Part model, mm, in its own coordinate system. Face numbers are marked on the shaded views. A direction names the side the tool comes from. Coordinates: 2 decimals unless noted, no trailing zeros. Order: outer loops, then holes, each group sorted by start corner. A loop starts at its lowest first (then second) coordinate and runs counter-clockwise, first axis right, second up.
1) Wall check: L1, parallel to Z at x = -18, y = 19.75; L2, parallel to X at y = 11.25, z = 20; L3, parallel to X at y = 20.1, z = -20. Give the ranges that are in metal, low to high.
2) Cut at C-C (z = 14). List the corners of the cut face in (x, y), and give its area (3 significant figures).
3) Pin check, flat tips, straight feed: pin 1 Ø2 at (y, z) = (18, -5.5) entering from +X; pin 2 Ø3.5 at (x, y) = (-0.5, 16) entering from -Z; pin 3 Ø4.5 at (x, z) = (18, 0.5) entering from +Y. Stop position of each tip, or through.
4) Mould opens along Z. For the marked faces 1, 2 and 3 say: +Z half, -Z half, draft (parallel to the pull), parting line (faces both ways), or undercut.
5) Cut at A-A (z = 1). List the corners of the cut face in (x, y), and give its area (3 significant figures).
6) Cut at D-D (x = 14.5). List the corners of the cut face in (y, z).
7) Cut at B-B (y = 9.25). List the corners of the cut face in (x, z), and give its area (3 significant figures).
8) Tool access for the marked faces 4, 5 and 6: list every direction of +Z, -Z, +X, -X, +Y, -Y with a clear straight run to the whole face (end or side of a thin tool).
```python
from build123d import *

# Parameters (mm, degrees)
ESQUISSE1_R             = 1.5
BOSS_EXTRU_1_DEPTH      = 20
ESQUISSE2_R             = 2.25
ESQUISSE2_R_2           = 1.5
BOSS_EXTRU_2_DEPTH      = 1.5
ESQUISSE6_W             = 7.215685205
ESQUISSE6_H             = 18.365547593
ESQUISSE6_W_2           = 15.795882497
ESQUISSE6_H_2           = 7.128539117
ESQUISSE6_W_3           = 6.98895005
ESQUISSE6_H_3           = 20.179428837
BOSS_EXTRU_3_DEPTH      = 14.8
ENL_V_MAT_EXTRU_1_DEPTH = 20
ENL_V_MAT_EXTRU_1_DRAFT = 10
ENL_V_MAT_EXTRU_2_DEPTH = 20
ENL_V_MAT_EXTRU_2_DRAFT = 7
ESQUISSE5_R             = 2.5
ENL_V_MAT_EXTRU_3_DEPTH = 18
CONG_4_R                = 1
CONG_5_R                = 1
CONG_6_R                = 1
CONG_7_R                = 1


with BuildPart() as part:
    # Esquisse1 → Boss.-Extru.1 (new body)
    with BuildSketch(Plane(origin=(0, 0, 0), x_dir=(1, 0, 0), z_dir=(0, 1, 0))):
        with BuildLine():
            Line((-19, 4.2), (-17.6, 4.2))
            ThreePointArc((-17.6, 4.2), (-15.832233047, 3.467766953), (-15.1, 1.7))
            Line((-15.1, 1.7), (-15.1, -1.7))
            ThreePointArc((-15.1, -1.7), (-15.832233047, -3.467766953), (-17.6, -4.2))
            Line((-17.6, -4.2), (-19, -4.2))
            ThreePointArc((-19, -4.2), (-20.767766953, -4.932233047), (-21.5, -6.7))
            Line((-21.5, -6.7), (-21.5, -20.5))
            Line((-21.5, -20.5), (-21.5, -23))
            Line((-21.5, -23), (-19, -23))
            Line((-19, -23), (-6.7, -23))
            ThreePointArc((-6.7, -23), (-4.932233047, -22.267766953), (-4.2, -20.5))
            Line((-4.2, -20.5), (-4.2, -19.1))
            ThreePointArc((-4.2, -19.1), (-3.467766953, -17.332233047), (-1.7, -16.6))
            Line((-1.7, -16.6), (1.7, -16.6))
            ThreePointArc((1.7, -16.6), (3.467766953, -17.332233047), (4.2, -19.1))
            Line((4.2, -19.1), (4.2, -20.5))
            ThreePointArc((4.2, -20.5), (4.932233047, -22.267766953), (6.7, -23))
            Line((6.7, -23), (19, -23))
            Line((19, -23), (21.5, -23))
            Line((21.5, -23), (21.5, -20.5))
            Line((21.5, -20.5), (21.5, -6.7))
            ThreePointArc((21.5, -6.7), (20.767766953, -4.932233047), (19, -4.2))
            Line((19, -4.2), (17.6, -4.2))
            ThreePointArc((17.6, -4.2), (15.832233047, -3.467766953), (15.1, -1.7))
            Line((15.1, -1.7), (15.1, 1.7))
            ThreePointArc((15.1, 1.7), (15.832233047, 3.467766953), (17.6, 4.2))
            Line((17.6, 4.2), (19, 4.2))
            ThreePointArc((19, 4.2), (20.767766953, 4.932233047), (21.5, 6.7))
            Line((21.5, 6.7), (21.5, 20.5))
            Line((21.5, 20.5), (21.5, 23))
            Line((21.5, 23), (19, 23))
            Line((19, 23), (6.7, 23))
            ThreePointArc((6.7, 23), (4.932233047, 22.267766953), (4.2, 20.5))
            Line((4.2, 20.5), (4.2, 19.1))
            ThreePointArc((4.2, 19.1), (3.467766953, 17.332233047), (1.7, 16.6))
            Line((1.7, 16.6), (-1.7, 16.6))
            ThreePointArc((-1.7, 16.6), (-3.467766953, 17.332233047), (-4.2, 19.1))
            Line((-4.2, 19.1), (-4.2, 20.5))
            ThreePointArc((-4.2, 20.5), (-4.932233047, 22.267766953), (-6.7, 23))
            Line((-6.7, 23), (-19, 23))
            Line((-19, 23), (-21.5, 23))
            Line((-21.5, 23), (-21.5, 20.5))
            Line((-21.5, 20.5), (-21.5, 6.7))
            ThreePointArc((-21.5, 6.7), (-20.767766953, 4.932233047), (-19, 4.2))
        make_face()
        with Locations(Location((-18, 20, 0), (0, 0, 270))):
            Circle(ESQUISSE1_R, mode=Mode.SUBTRACT)
        with Locations(Location((18, 20, 0), (0, 0, 270))):
            Circle(ESQUISSE1_R, mode=Mode.SUBTRACT)
        with Locations(Location((18, -20, 0), (0, 0, 270))):
            Circle(ESQUISSE1_R, mode=Mode.SUBTRACT)
        with Locations(Location((-18, -20, 0), (0, 0, 270))):
            Circle(ESQUISSE1_R, mode=Mode.SUBTRACT)
    extrude(amount=BOSS_EXTRU_1_DEPTH)

    # Esquisse2 → Boss.-Extru.2 (add)
    # profile 1 of 4: a face of its own
    with BuildSketch(Plane(origin=(0, 20, 0), x_dir=(1, 0, 0), z_dir=(0, 1, 0))):
        with Locations(Location((-18, 20, 0), (0, 0, 270))):
            Circle(ESQUISSE2_R)
        with Locations(Location((-18, 20, 0), (0, 0, 270))):
            Circle(ESQUISSE2_R_2, mode=Mode.SUBTRACT)
    # profile 2 of 4: a face of its own
    with BuildSketch(Plane(origin=(0, 20, 0), x_dir=(1, 0, 0), z_dir=(0, 1, 0))):
        with Locations(Location((18, 20, 0), (0, 0, 270))):
            Circle(ESQUISSE2_R)
        with Locations(Location((18, 20, 0), (0, 0, 270))):
            Circle(ESQUISSE2_R_2, mode=Mode.SUBTRACT)
    # profile 3 of 4: a face of its own
    with BuildSketch(Plane(origin=(0, 20, 0), x_dir=(1, 0, 0), z_dir=(0, 1, 0))):
        with Locations(Location((18, -20, 0), (0, 0, 270))):
            Circle(ESQUISSE2_R)
        with Locations(Location((18, -20, 0), (0, 0, 270))):
            Circle(ESQUISSE2_R_2, mode=Mode.SUBTRACT)
    # profile 4 of 4: a face of its own
    with BuildSketch(Plane(origin=(0, 20, 0), x_dir=(1, 0, 0), z_dir=(0, 1, 0))):
        with Locations(Location((-18, -20, 0), (0, 0, 270))):
            Circle(ESQUISSE2_R)
        with Locations(Location((-18, -20, 0), (0, 0, 270))):
            Circle(ESQUISSE2_R_2, mode=Mode.SUBTRACT)
    extrude(amount=BOSS_EXTRU_2_DEPTH)

    # Esquisse6 → Boss.-Extru.3 (add)
    with BuildSketch(Plane.XZ):
        with Locations((-17.892157398, 0.340102734)):
            Rectangle(ESQUISSE6_W, ESQUISSE6_H)
        with Locations((-0.491259504, 19.435730441)):
            Rectangle(ESQUISSE6_W_2, ESQUISSE6_H_2)
        with Locations((18.005524975, 1.247043355)):
            Rectangle(ESQUISSE6_W_3, ESQUISSE6_H_3)
        with BuildLine():
            Line((-4.2, -19.1), (-4.2, -20.5))
            ThreePointArc((-4.2, -20.5), (-4.932233047, -22.267766953), (-6.7, -23))
            Line((-6.7, -23), (8.691514293, -23))
            Line((8.691514293, -23), (8.691514293, -16.6))
            Line((8.691514293, -16.6), (-1.7, -16.6))
            ThreePointArc((-1.7, -16.6), (-3.467766953, -17.332233047), (-4.2, -19.1))
        make_face()
    extrude(amount=-BOSS_EXTRU_3_DEPTH)


with BuildPart() as enl_v_mat_extru_1_tool:
    # Esquisse3 → Enlèv. mat.-Extru.1 (with draft: the straight prism first)
    with BuildSketch(Plane(origin=(0, 20, 0), x_dir=(1, 0, 0), z_dir=(0, 1, 0))):
        with BuildLine():
            ThreePointArc((-4.5, 7.5), (-6.621320344, 6.621320344), (-7.5, 4.5))
            Line((-7.5, 4.5), (-7.5, -4.5))
            ThreePointArc((-7.5, -4.5), (-6.621320344, -6.621320344), (-4.5, -7.5))
            Line((-4.5, -7.5), (4.5, -7.5))
            ThreePointArc((4.5, -7.5), (6.621320344, -6.621320344), (7.5, -4.5))
            Line((7.5, -4.5), (7.5, 4.5))
            ThreePointArc((7.5, 4.5), (6.621320344, 6.621320344), (4.5, 7.5))
            Line((4.5, 7.5), (-4.5, 7.5))
        make_face()
    extrude(amount=-ENL_V_MAT_EXTRU_1_DEPTH)
    # Enlèv. mat.-Extru.1: the draft: its side faces are tilted about the plane it starts from
    enl_v_mat_extru_1_sides = [enl_v_mat_extru_1_tool.faces().sort_by_distance(p)[0] for p in [
        (-6.621320344, 10, -6.621320344),
        (-7.5, 10, 0),
        (-6.621320344, 10, 6.621320344),
        (0, 10, 7.5),
        (6.621320344, 10, 6.621320344),
        (7.5, 10, 0),
        (6.621320344, 10, -6.621320344),
        (0, 10, -7.5),
    ]]
    draft(enl_v_mat_extru_1_sides, Plane(origin=(0, 20, 0), x_dir=(1, 0, 0), z_dir=(0, 1, 0)), ENL_V_MAT_EXTRU_1_DRAFT)


with BuildPart() as part_1:
    add(part.part)

    # Enlèv. mat.-Extru.1: cut by enl_v_mat_extru_1_tool
    add(enl_v_mat_extru_1_tool.part, mode=Mode.SUBTRACT)


with BuildPart() as enl_v_mat_extru_2_tool:
    # Esquisse4 → Enlèv. mat.-Extru.2 (with draft: the straight prism first)
    with BuildSketch(Plane(origin=(0, 20, 0), x_dir=(1, 0, 0), z_dir=(0, 1, 0))):
        with BuildLine():
            ThreePointArc((6.1, 20), (5.746446609, 19.853553391), (5.6, 19.5))
            Line((5.6, 19.5), (5.6, 16.7))
            ThreePointArc((5.6, 16.7), (5.746446609, 16.346446609), (6.1, 16.2))
            Line((6.1, 16.2), (10.9, 16.2))
            ThreePointArc((10.9, 16.2), (11.253553391, 16.346446609), (11.4, 16.7))
            Line((11.4, 16.7), (11.4, 19.5))
            ThreePointArc((11.4, 19.5), (11.253553391, 19.853553391), (10.9, 20))
            Line((10.9, 20), (6.1, 20))
        make_face()
    extrude(amount=-ENL_V_MAT_EXTRU_2_DEPTH)
    # Enlèv. mat.-Extru.2: the draft: its side faces are tilted about the plane it starts from
    enl_v_mat_extru_2_sides = [enl_v_mat_extru_2_tool.faces().sort_by_distance(p)[0] for p in [
        (11.253553391, 10, -19.853553391),
        (8.5, 10, -20),
        (5.746446609, 10, -19.853553391),
        (5.6, 10, -18.1),
        (5.746446609, 10, -16.346446609),
        (8.5, 10, -16.2),
        (11.253553391, 10, -16.346446609),
        (11.4, 10, -18.1),
    ]]
    draft(enl_v_mat_extru_2_sides, Plane(origin=(0, 20, 0), x_dir=(1, 0, 0), z_dir=(0, 1, 0)), ENL_V_MAT_EXTRU_2_DRAFT)


with BuildPart() as part_2:
    add(part_1.part)

    # Enlèv. mat.-Extru.2: cut by enl_v_mat_extru_2_tool
    add(enl_v_mat_extru_2_tool.part, mode=Mode.SUBTRACT)

    # Esquisse5 → Enlèv. mat.-Extru.3 (cut)
    with BuildSketch(Plane.XZ):
        with Locations(Location((-18, 20, 0), (0, 0, 270))):
            Circle(ESQUISSE5_R)
        with Locations(Location((18, 20, 0), (0, 0, 270))):
            Circle(ESQUISSE5_R)
        with Locations(Location((18, -20, 0), (0, 0, 270))):
            Circle(ESQUISSE5_R)
        with Locations(Location((-18, -20, 0), (0, 0, 270))):
            Circle(ESQUISSE5_R)
    extrude(amount=-ENL_V_MAT_EXTRU_3_DEPTH, mode=Mode.SUBTRACT)

    # Congé4
    cong_4_edges = [part_2.edges().sort_by_distance(p)[0] for p in [
        (-21.5, 14.8, 0),
    ]]
    fillet(cong_4_edges, radius=CONG_4_R)

    # Congé5
    cong_5_edges = [part_2.edges().sort_by_distance(p)[0] for p in [
        (0, 14.8, 23),
    ]]
    fillet(cong_5_edges, radius=CONG_5_R)

    # Congé6
    cong_6_edges = [part_2.edges().sort_by_distance(p)[0] for p in [
        (21.5, 14.8, 0),
    ]]
    fillet(cong_6_edges, radius=CONG_6_R)

    # Congé7
    cong_7_edges = [part_2.edges().sort_by_distance(p)[0] for p in [
        (0, 14.8, -23),
    ]]
    fillet(cong_7_edges, radius=CONG_7_R)


solid = part_2.part
```
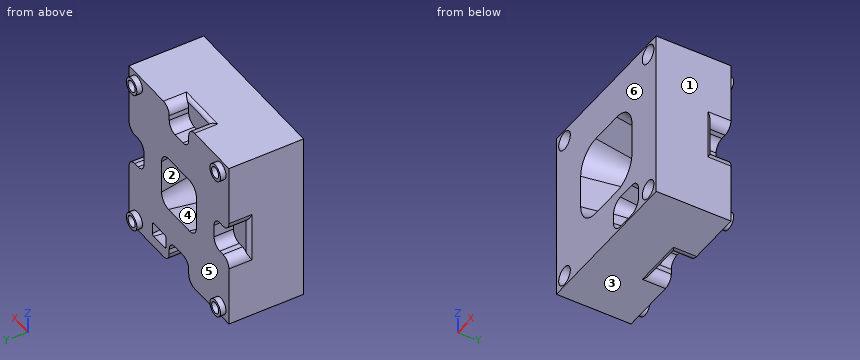
Geometry check:
1. L1: z = -23 to -21.5, -18.5 to -4.2, 4.2 to 18.5, 21.5 to 23
1. L2: x = -21.5 to -20.5, -15.5 to 15.5, 20.5 to 21.5
1. L3: x = -20.25 to -19.5, -16.5 to -15.75, 15.75 to 16.5, 19.5 to 20.25
2. outline: (-21.5, 0) - (21.5, 0) - (21.5, 20) - (-21.5, 20) - close
2. area: 860 mm2
3. pin 1: stops at x = 21.49
3. pin 2: stops at z = -22.89
3. pin 3: stops at y = 14.8
4. face 1: draft
4. face 2: undercut
4. face 3: -Z half
5. outline: (-21.5, 0) - (-11.03, 0) - (-7.5, 20) - (-15.1, 20) - (-15.1, 14.8) - (-20.5, 14.8) arc R1 ccw to (-21.5, 13.8) - close; (7.5, 20) - (11.03, 0) - (21.5, 0) - (21.5, 13.8) arc R1 ccw to (20.5, 14.8) - (15.1, 14.8) - (15.1, 20) - close
5. area: 422 mm2
6. outline: (0, -23) - (20, -23) - (20, 23) - (0, 23) - close
7. outline: (-21.5, -23) - (21.5, -23) - (21.5, 23) - (-21.5, 23) - close; hole circle Ø5 at (-18, -20); hole circle Ø5 at (-18, 20); hole (-9.4, -4.5) arc R4.9 ccw to (-4.5, -9.4) - (4.5, -9.4) arc R4.9 ccw to (9.4, -4.5) - (9.4, 4.5) arc R4.9 ccw to (4.5, 9.4) - (-4.5, 9.4) arc R4.9 ccw to (-9.4, 4.5) - close; hole (4.28, -19.5) arc R1.82 ccw to (6.1, -21.32) - (10.9, -21.32) arc R1.82 ccw to (12.72, -19.5) - (12.72, -16.7) arc R1.82 ccw to (10.9, -14.88) - (6.1, -14.88) arc R1.82 ccw to (4.28, -16.7) - close; hole circle Ø5 at (18, -20); hole circle Ø5 at (18, 20)
7. area: 1,520 mm2
8. face 4: -Y
8. face 5: +Y
8. face 6: +Z, -Z, +X, -X, -Y
